```python
from build123d import *

# Parameters (mm, degrees)
SKETCH10_W                = 6
SKETCH10_H                = 6
RACK_BAR_DEPTH            = 11.5
RACK_ROOT_STEP_DEPTH      = 13.257650672
RACK_ROOT_STEP_DEPTH_BACK = 13.257650672
SKETCH12_W                = 2.75
SKETCH12_H                = 24
RACK_TEETH_DEPTH          = 3
SKETCH15_R                = 1.001320398
CUT_EXTRUDE2_DEPTH        = 4.5


with BuildPart() as part:
    # Sketch10 → RACK_BAR (new, symmetric)
    with BuildSketch(Plane.XY):
        Rectangle(SKETCH10_W, SKETCH10_H)
    extrude(amount=RACK_BAR_DEPTH, both=True)

    # Sketch12 → RACK_ROOT_STEP (cut, two sides: drawn at the far end of the back side and taken through both)
    with BuildSketch(Plane(origin=(0, 0, 0), x_dir=(1, 0, 0), z_dir=(0, 1, 0)).offset(-RACK_ROOT_STEP_DEPTH_BACK)):
        with Locations((2.125, 0)):
            Rectangle(SKETCH12_W, SKETCH12_H)
    extrude(amount=RACK_ROOT_STEP_DEPTH + RACK_ROOT_STEP_DEPTH_BACK, mode=Mode.SUBTRACT)

    # Sketch13 → RACK_TEETH (add, symmetric)
    with BuildSketch(Plane(origin=(0, 0, 0), x_dir=(1, 0, 0), z_dir=(0, 1, 0))):
        Polygon((0.5, 1.3314), (3, 0.4214), (3, -0.4214), (0.5, -1.3314), align=None)
        Polygon((0.5, 4.473), (3, 3.563), (3, 2.7202), (0.5, 1.8102), align=None)
        Polygon((0.5, -1.8102), (3, -2.7202), (3, -3.563), (0.5, -4.473), align=None)
        Polygon((0.5, 7.6146), (3, 6.7046), (3, 5.8618), (0.5, 4.9518), align=None)
        Polygon((0.5, -4.9518), (3, -5.8618), (3, -6.7046), (0.5, -7.6146), align=None)
        Polygon((0.5, 10.7562), (3, 9.8462), (3, 9.0034), (0.5, 8.0934), align=None)
        Polygon((0.5, -8.0934), (3, -9.0034), (3, -9.8462), (0.5, -10.7562), align=None)
    extrude(amount=RACK_TEETH_DEPTH, both=True)

    # Sketch15 → Cut-Extrude2 (cut)
    with BuildSketch(Plane(origin=(0, 0, -11.5), x_dir=(-1, 0, 0), z_dir=(0, 0, -1))):
        with Locations((1.25, 0)):
            Circle(SKETCH15_R)
    extrude(amount=-CUT_EXTRUDE2_DEPTH, mode=Mode.SUBTRACT)


solid = part.part
```
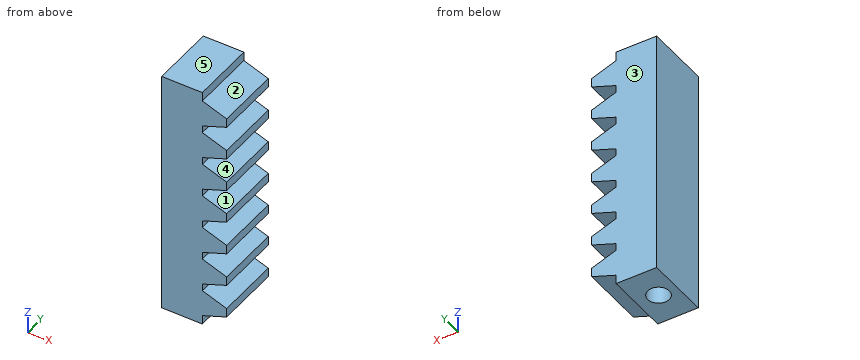
Read the model definition and answer for the solid it produces. Units are mm, in the model's axes. Face numbers are marked on the shaded views. A direction names the side the tool comes from. Coordinates: 2 decimals unless noted, no trailing zeros. Write each loop counter-clockwise with the first axis right and the second up, starting at its lowest first coordinate (ties: lowest second). Pieces come first, ordered by that corner, then holes. Notation, with made-up numbers: (12.5, 79.25) -> (42.5, 79.25) arc R31 ccw to (42.5, 110.25) -> close; hole circle Ø1 at (78, 55). An arc over 180 degrees is marked (long way). Return JSON: item names as keys, results as strings.
1. A tool of negligible diameter and unlimited length cuts with its end or side. For the marked faces 1 and 2, from which of +Z, -Z, +X, -X, +Y, -Y can it reach the whole face along a straight path? Write none if from no direction.
Found:
{"face 1": "+X, +Y, -Y", "face 2": "+Z, +X, +Y, -Y"}
2. This flat-tipped pin is pushed along its axis until it touches: P1, Ø1, axis at x = -1.5, y = 0, coming from the -Z side. Where does it stop, or does it pass through?
Found:
{"P1": "z = -7"}
3. A cutting plane is placed at C-C (z = 8.75). Determine the outline of the cut face in (x, y), and give its area (3 significant figures).
Found:
{"outline": "(-3, -3) -> (2.3, -3) -> (2.3, 3) -> (-3, 3) -> close", "area": "31.8 mm2"}
4. A cutting plane is placed at D-D (z = 2.25). Determine the outline of the cut face in (x, y), and give its area (3 significant figures).
Found:
{"outline": "(-3, -3) -> (1.71, -3) -> (1.71, 3) -> (-3, 3) -> close", "area": "28.2 mm2"}
5. Determine the mould class of the marked faces 3, 4 and 5 for opening direction Z: pulls with the +Z half, pulls with the -Z half, needs draft (parallel to the pull), parting line crosses it, or undercut.
Found:
{"face 3": "needs draft", "face 4": "undercut", "face 5": "pulls with the +Z half"}
6. A cutting plane is placed at A-A (x = -1.25). Determine the outline of the cut face in (y, z), and give its area (3 significant figures).
Found:
{"outline": "(-3, -11.5) -> (-1, -11.5) -> (-1, -7) -> (1, -7) -> (1, -11.5) -> (3, -11.5) -> (3, 11.5) -> (-3, 11.5) -> close", "area": "129 mm2"}
7. Find the intervals of material crossed by line 1 along Y through (x, z) = (-1.25, -9.6); line 2 along X through (y, z) = (2.75, 8), in increasing order. Write a range as from..to.
Found:
{"line 1": "-3..-1, 1..3", "line 2": "-3..0.75"}
